Part print with two shaded views. Sizes in mm from the minimum x, y, z corner. Coordinates: 2 decimals unless noted, no trailing zeros. Write each loop counter-clockwise with the first axis right and the second up, starting at its lowest first coordinate (ties: lowest second). Pieces come first, ordered by that corner, then holes. Notation, with made-up numbers: (71, 49) - (83, 49) arc R24 ccw to (83, 73) - close; hole circle Ø8 at (-16.75, 61.25). An arc over 180 degrees is marked (long way). Answer in a Markdown table with one row per item. Add a question column.
Q1. Band-saw the part on B-B (x = 11). List the corners of the cut face in (y, z), and give its area (3 significant figures).
Q2. Band-saw the part on A-A (z = 3.5). List the corners of the cut face in (x, y), and give its area (3 significant figures).
Q3. Drill centre lines: line 1 along X through (y, z) = (6, 5.25); line 2 along Z through (x, y) = (36.5, 3.75); line 3 along Z through (x, y) = (24.5, 5). Where is each one in solid material? Low to high. Write a range as from..to.
Q4. Pin check, flat tips, straight feed: pin 1 (1.5 mm diameter, centred on x = 60, z = 2.5, fed in from -Y); pin 2 (1 mm diameter, centred on x = 55.5, y = 6, fed in from -Z); pin 3 (1 mm diameter, centred on x = 63, z = 5.5, fed in from +Y). Stop position of each tip, or through.
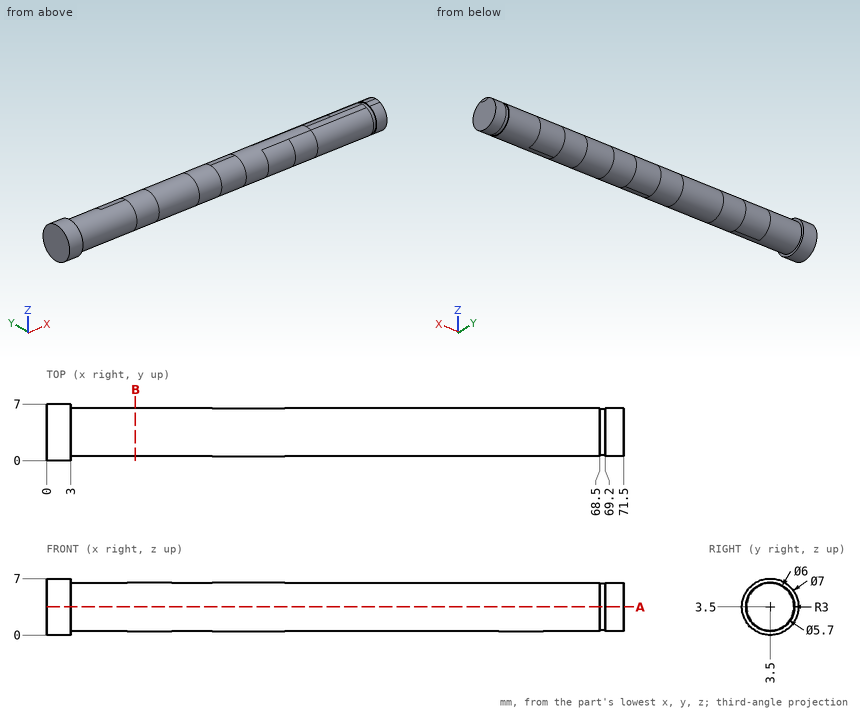
Checked values:
| question | item | result |
|---|---|---|
| 1 | outline | circle Ø6 at (3.5, 3.5) |
| 1 | area | 28.3 mm² |
| 2 | outline | (0, 0) - (3, 0) - (3, 0.5) - (68.5, 0.5) - (68.5, 0.65) - (69.2, 0.65) - (69.2, 0.5) - (71.5, 0.5) - (71.5, 6.5) - (69.2, 6.5) - (69.2, 6.35) - (68.5, 6.35) - (68.5, 6.5) - (3, 6.5) - (3, 7) - (0, 7) - close |
| 2 | area | 432 mm² |
| 3 | line 1 | x = 0..3 |
| 3 | line 2 | z = 0.51..6.49 |
| 3 | line 3 | z = 0.9..6.1 |
| 4 | pin 1 | stops at y = 0.51 |
| 4 | pin 2 | stops at z = 1.26 |
| 4 | pin 3 | stops at y = 6.1 |
